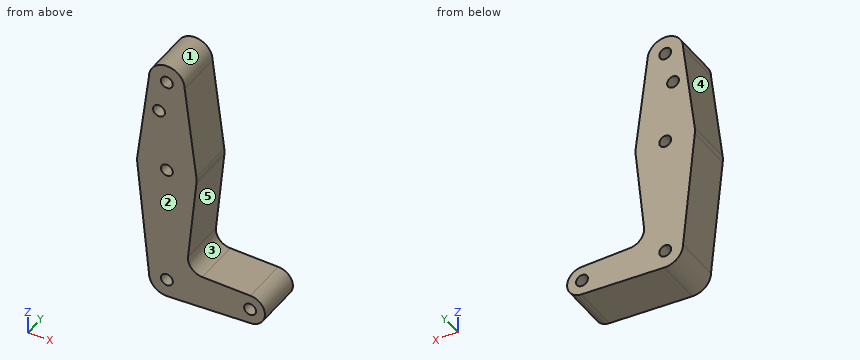
from build123d import *

# Parameters (mm, degrees)
F0_R     = 3.175
F1_DEPTH = 25.4


with BuildPart() as f1:
    # F0 (on Front) → F1 (new body)
    with BuildSketch(Plane.XZ):
        with BuildLine():
            ThreePointArc((9.525, 0), (6.7351920908, 6.7351920908), (0, 9.525))
            ThreePointArc((0, 9.525), (-6.7351920908, 6.7351920908), (-9.525, 0))
            ThreePointArc((-9.525, 0), (-6.6138274083, -6.8544082176), (0.3401783754, -9.5189234514))
            ThreePointArc((0.3401783754, -9.5189234514), (6.8544082176, -6.6138274083), (9.525, 0))
        make_face()
        with BuildLine():
            ThreePointArc((3.175, 0), (-2.2450640303, -2.2450640303), (0, 3.175))
            ThreePointArc((0, 3.175), (2.2450640303, 2.2450640303), (3.175, 0))
        make_face(mode=Mode.SUBTRACT)
        with BuildLine():
            ThreePointArc((-9.525, 0), (-6.7351920908, 6.7351920908), (0, 9.525))
            Line((0, 9.525), (0, 47.625))
            ThreePointArc((0, 47.625), (-10.644756084, 51.722700101), (-15.7942028036, 61.9003804205))
            Line((-15.7942028036, 61.9003804205), (-9.525, 0))
        make_face()
        with BuildLine():
            Line((0, 47.625), (0, 9.525))
            ThreePointArc((0, 9.525), (6.7351920908, 6.7351920908), (9.525, 0))
            ThreePointArc((9.525, 0), (6.8544082176, -6.6138274083), (0.3401783754, -9.5189234514))
            Line((0.3401783754, -9.5189234514), (44.7334821429, -7.9324362036))
            ThreePointArc((44.7334821429, -7.9324362036), (36.5127422872, -0.0620181515), (44.6094941417, 7.9358974205))
            Line((44.6094941417, 7.9358974205), (18.9338924558, 8.8505270449))
            ThreePointArc((18.9338924558, 8.8505270449), (13.2248772537, 11.5706407269), (11.3071823287, 17.5967770675))
            Line((11.3071823287, 17.5967770675), (15.7942028036, 61.9003804205))
            ThreePointArc((15.7942028036, 61.9003804205), (10.644756084, 51.722700101), (0, 47.625))
        make_face()
        with BuildLine():
            ThreePointArc((-15.7942028036, 61.9003804205), (-10.644756084, 51.722700101), (0, 47.625))
            Line((0, 47.625), (0, 60.325))
            ThreePointArc((0, 60.325), (-3.175, 63.5), (0, 66.675))
            Line((0, 66.675), (0, 79.375))
            ThreePointArc((0, 79.375), (-10.4912828548, 75.4142187767), (-15.7474569047, 65.5082893304))
            ThreePointArc((-15.7474569047, 65.5082893304), (-15.873667691, 63.7056672947), (-15.7942028036, 61.9003804205))
        make_face()
        with BuildLine():
            Line((0, 60.325), (0, 47.625))
            ThreePointArc((0, 47.625), (10.644756084, 51.722700101), (15.7942028036, 61.9003804205))
            ThreePointArc((15.7942028036, 61.9003804205), (15.8547878338, 62.6991705884), (15.875, 63.5))
            ThreePointArc((15.875, 63.5), (15.8430821396, 64.5061676396), (15.7474569047, 65.5082893304))
            ThreePointArc((15.7474569047, 65.5082893304), (10.4912828548, 75.4142187767), (0, 79.375))
            Line((0, 79.375), (0, 66.675))
            ThreePointArc((0, 66.675), (2.2450640303, 65.7450640303), (3.175, 63.5))
            ThreePointArc((3.175, 63.5), (2.2450640303, 61.2549359697), (0, 60.325))
        make_face()
        with BuildLine():
            Line((-9.525, 114.3), (-15.7474569047, 65.5082893304))
            ThreePointArc((-15.7474569047, 65.5082893304), (-10.4912828548, 75.4142187767), (0, 79.375))
            Line((0, 79.375), (0, 104.775))
            ThreePointArc((0, 104.775), (-6.7351920908, 107.5648079092), (-9.525, 114.3))
        make_face()
        with Locations((-4.1781016625, 96.3086113334)):
            Circle(F0_R, mode=Mode.SUBTRACT)
        with BuildLine():
            ThreePointArc((44.6094941417, 7.9358974205), (36.5127422872, -0.0620181515), (44.7334821429, -7.9324362036))
            ThreePointArc((44.7334821429, -7.9324362036), (50.1620069047, -5.5115227815), (52.3875, 0))
            ThreePointArc((52.3875, 0), (50.1187693109, 5.5559842287), (44.6094941417, 7.9358974205))
        make_face()
        with Locations((44.45, 0)):
            Circle(F0_R, mode=Mode.SUBTRACT)
        with BuildLine():
            Line((0, 104.775), (0, 79.375))
            ThreePointArc((0, 79.375), (10.4912828548, 75.4142187767), (15.7474569047, 65.5082893304))
            Line((15.7474569047, 65.5082893304), (9.525, 114.3))
            ThreePointArc((9.525, 114.3), (6.7351920908, 107.5648079092), (0, 104.775))
        make_face()
        with BuildLine():
            ThreePointArc((9.525, 114.3), (0, 123.825), (-9.525, 114.3))
            ThreePointArc((-9.525, 114.3), (-6.7351920908, 107.5648079092), (0, 104.775))
            ThreePointArc((0, 104.775), (6.7351920908, 107.5648079092), (9.525, 114.3))
        make_face()
        with BuildLine():
            ThreePointArc((3.175, 114.3), (2.2450640303, 112.0549359697), (0, 111.125))
            ThreePointArc((0, 111.125), (-2.2450640303, 116.5450640303), (3.175, 114.3))
        make_face(mode=Mode.SUBTRACT)
    extrude(amount=F1_DEPTH)


solid = f1.part
CAD build for the part. Positions are in the model's coordinates, mm. Face numbers are marked on the shaded views. A direction names the side the tool comes from. Give positions to 0.01 mm unless a question says otherwise; leave off trailing zeros. Write each loop counter-clockwise with the first axis right and the second up, starting at its lowest first coordinate (ties: lowest second). Pieces come first, ordered by that corner, then holes. Notation, with made-up numbers: M 7,74.25 L 27,74.25 A20 ccw 27,79.25 Z; hole C 44,4.25 d2. An arc over 180 degrees is marked long. Put each result on its own line as item: value. Start each with the question number.
(1) Band-saw the part on A-A, the plane y = -15.25. Give the number of separate pieces and of enclosed holes in the cut face, and give its area (3 significant figures).
(2) Mould opens along Z. For the marked faces 1, 2 and 3 say: +Z half, -Z half, draft (parallel to the pull), parting line (faces both ways), or undercut.
(3) Probe L1, parallel to Z at x = 44.45, y = -10 (3 decimals); L2, parallel to Z at x = 0, y = -5.5 (3 decimals); L3, parallel to X at y = -11, z = -2. List the from-to ranges inside material, lowest first.
(4) Flat gauge pins, fed straight in: pin 1 Ø10 at (x, z) = (0, 114.3) entering from +Y; pin 2 Ø3 at (y, z) = (-18, 107.5) entering from +X; pin 3 Ø3 at (y, z) = (-13.5, 18) entering from +X; pin 4 Ø1.5 at (x, y) = (44, -22.5) entering from -Z. Where does each tip first touch, or does it go through?
(5) Band-saw the part on C-C, the plane z = 47.5. Write the cut outline in (x, y), and give its area (3 significant figures).
(6) Which spindle directions (+Z, -Z, +X, -X, +Y, -Y) get a long thin tool onto all of the face, cutting with end or side? Do the marked faces 4 and 5. Say none if no direction does.
(7) Band-saw the part on B-B, the plane x = -6. Write the cut outline in (y, z).
Response values:
1. separate pieces: 1
1. enclosed holes: 5
1. area: 3,770 mm2
2. face 1: +Z half
2. face 2: draft
2. face 3: undercut
3. L1: z = -7.943 to -3.175, 3.175 to 7.942
3. L2: z = -9.525 to -3.175, 3.175 to 60.325, 66.675 to 111.125, 117.475 to 123.825
3. L3: x = -9.31 to -2.47, 2.47 to 41.98, 46.92 to 52.13
4. pin 1: stops at y = 0
4. pin 2: stops at x = 10.58
4. pin 3: stops at x = 11.5
4. pin 4: stops at z = -7.99
5. outline: M -14.34,-25.4 L 14.34,-25.4 L 14.34,0 L -14.34,0 Z
5. area: 728 mm2
6. face 4: +Z, -X, +Y, -Y
6. face 5: +X, +Y, -Y
7. outline: M -25.4,-7.4 L 0,-7.4 L 0,93.71 L -25.4,93.71 Z; M -25.4,98.91 L 0,98.91 L 0,121.7 L -25.4,121.7 Z
